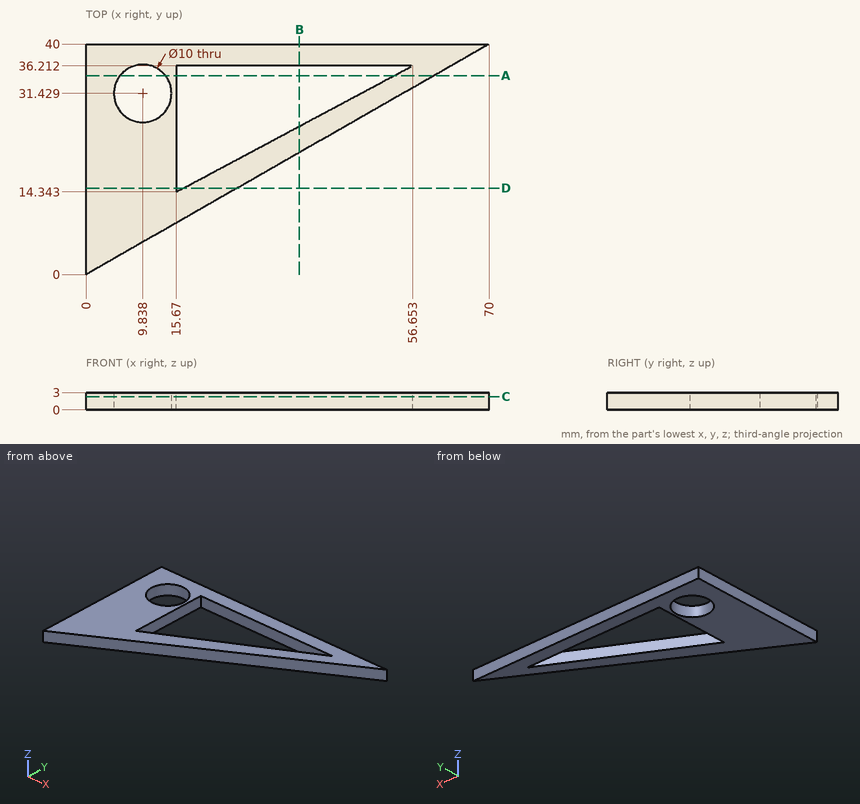
Drawing for the job (mm, zero at the part's lowest x, y, z). Round coordinates to 2 decimals unless told otherwise and drop trailing zeros. Loops run counter-clockwise (first coordinate to the right, second up) from the corner with the lowest first, then second, coordinate; pieces in that order, holes last. Notation, with made-up numbers: M 65,33.25 L 110,33.25 A11 cw 110,38.25 Z; hole C 77.5,62 d8. An arc over 180 degrees is marked long. Use a Markdown table: item, result. Add a question column.
(1) Cut at B-B (x = 37). Give the cut face in (y, z) (1 decimal).
(2) Cut at A-A (y = 34.5). Give the cut face in (x, z) (1 decimal).
(3) Cut at D-D (y = 15). Give the cut face in (x, z).
(4) Drill centre lines: line 1 (X direction, y = 28, z = 2.75) (1 decimal); line 2 (Y direction, x = 8, z = 1.2); line 3 (Y direction, x = 21, z = 1.2) (1 decimal). Where is each one in solid material? Low to high.
(5) Cut at C-C (z = 2.3). Give the cut face in (x, y).
Geometry says:
| question | item | result |
|---|---|---|
| 1 | outline | M 21.1,0 L 25.7,0 L 25.7,3 L 21.1,3 Z; M 36.2,0 L 40,0 L 40,3 L 36.2,3 Z |
| 2 | outline | M 0,0 L 5.9,0 L 5.9,3 L 0,3 Z; M 13.8,0 L 15.7,0 L 15.7,3 L 13.8,3 Z; M 53.4,0 L 60.4,0 L 60.4,3 L 53.4,3 Z |
| 3 | outline | M 0,0 L 15.67,0 L 15.67,3 L 0,3 Z; M 16.9,0 L 26.25,0 L 26.25,3 L 16.9,3 Z |
| 4 | line 1 | x = 0 to 6.2, 13.5 to 15.7, 41.3 to 49 |
| 4 | line 2 | y = 4.57 to 26.78, 36.08 to 40 |
| 4 | line 3 | y = 12 to 17.2, 36.2 to 40 |
| 5 | outline | M 0,0 L 70,40 L 0,40 Z; hole C 9.84,31.43 d10; hole M 15.67,14.34 L 56.65,36.21 L 15.67,36.21 Z |
